Build history of the part. All positions in model axes, mm. Face numbers are marked on the shaded views. A direction names the side the tool comes from. Round coordinates to 2 decimals unless told otherwise and drop trailing zeros. Order: outer loops, then holes, each group sorted by start corner. A loop starts at its lowest first (then second) coordinate and runs counter-clockwise, first axis right, second up. Notation, with made-up numbers: (34.25, -21) - (66.25, -21) arc R14 ccw to (66.25, 6) - close; hole circle Ø3 at (81, 9). An arc over 180 degrees is marked (long way). Write each question's results on one line, items separated by ' | '. Start each with the question number.
```python
from build123d import *
from OCP.BRepFilletAPI import BRepFilletAPI_MakeChamfer

# Parameters (mm, degrees)
BOSS_EXTRUDE1_DEPTH             = 2
BOSS_EXTRUDE2_REACH             = 40.8
SKETCH2_W                       = 18.81765306
SKETCH2_H                       = 6
BOSS_EXTRUDE2_DIRECTION_2_DEPTH = 10
CUT_EXTRUDE1_DEPTH              = 8
CUT_EXTRUDE2_DEPTH              = 38.936459462
CUT_EXTRUDE2_DEPTH_BACK         = 38.936459462
SKETCH4_W                       = 8
SKETCH4_H                       = 2
CHAMFER1_SIZE                   = 2
CHAMFER2_SIZE                   = 10
CHAMFER2_SIZE2                  = 5.773502692
FILLET1_R                       = 20
BOSS_EXTRUDE3_START             = -6
SKETCH5_W                       = 10
SKETCH5_H                       = 1.6
BOSS_EXTRUDE3_DEPTH             = 12


with BuildPart() as part:
    # Sketch1 → Boss-Extrude1 (new, symmetric)
    with BuildSketch(Plane(origin=(0, 0, 0), x_dir=(1, 0, 0), z_dir=(0, 1, 0))):
        Polygon((-8.25, 0), (0, 0), (0, -1.2), (-9.40882653, -1.2), (-9.962319737, 14.649971666), (-19.979363266, 32), (-18.59372262, 32), (-8.773492451, 14.990862405), align=None)
    boss_extrude1 = extrude(amount=BOSS_EXTRUDE1_DEPTH, both=True)

    # Mirror1: Boss-Extrude1 across plane
    add(boss_extrude1.mirror(Plane(origin=(0, 2, 0), x_dir=(0, 0, 1), z_dir=(-1, 0, 0))))

    # Boss-Extrude2: up to this face of the body (flat: up to its plane)
    boss_extrude2_end = Plane(part.part.faces().sort_by_distance((0, 0, 0))[0])
    # Sketch2 → Boss-Extrude2 (add, up to the picked face)
    with BuildSketch(Plane.XY.offset(1.2), mode=Mode.PRIVATE) as boss_extrude2_sk1:
        with Locations((0, -1)):
            Rectangle(SKETCH2_W, SKETCH2_H)
    boss_extrude2_tool1 = split(extrude(boss_extrude2_sk1.sketch, amount=-BOSS_EXTRUDE2_REACH, mode=Mode.PRIVATE), bisect_by=boss_extrude2_end, keep=Keep.BOTH, mode=Mode.PRIVATE)
    add(boss_extrude2_tool1.solids().sort_by(Axis((0, -1, 1.2), (0, 0, -1)))[0])

    # Sketch2 → Boss-Extrude2 direction 2 (add)
    with BuildSketch(Plane.XY.offset(1.2)):
        with Locations((0, -1)):
            Rectangle(SKETCH2_W, SKETCH2_H)
    extrude(amount=BOSS_EXTRUDE2_DIRECTION_2_DEPTH)

    # Sketch3 → Cut-Extrude1 (cut)
    with BuildSketch(Plane.XY.offset(11.2)):
        with BuildLine():
            Line((-1.5, 1.826658805), (-1.5, 2))
            Line((-1.5, 2), (1.5, 2))
            Line((1.5, 2), (1.5, 1.826658805))
            ThreePointArc((1.5, 1.826658805), (3.2, -1), (1.5, -3.826658805))
            Line((1.5, -3.826658805), (1.5, -4))
            Line((1.5, -4), (-1.5, -4))
            Line((-1.5, -4), (-1.5, -3.826658805))
            ThreePointArc((-1.5, -3.826658805), (-3.2, -1), (-1.5, 1.826658805))
        make_face()
    extrude(amount=-CUT_EXTRUDE1_DEPTH, mode=Mode.SUBTRACT)

    # Sketch4 → Cut-Extrude2 (cut, two sides: drawn at the far end of the back side and taken through both)
    with BuildSketch(Plane(origin=(0, 0, 0), x_dir=(1, 0, 0), z_dir=(0, 1, 0)).offset(-CUT_EXTRUDE2_DEPTH_BACK)):
        with Locations((0, -4.2)):
            Rectangle(SKETCH4_W, SKETCH4_H)
    extrude(amount=CUT_EXTRUDE2_DEPTH + CUT_EXTRUDE2_DEPTH_BACK, mode=Mode.SUBTRACT)

    # Chamfer1
    chamfer1_edges = [part.edges().sort_by_distance(p)[0] for p in [
        (8.829413265, -2, 0),
        (-8.829413265, -2, 0),
    ]]
    chamfer(chamfer1_edges, length=CHAMFER1_SIZE - 0.0001)  # a hair under: the kernel refuses the full size

    # Chamfer2: one chamfer whose edges measure the first distance from different faces: ONE call of the kernel's chamfer builder (chamfer() names one face for all edges)
    chamfer2_edges_1 = [part.edges().sort_by_distance(p)[0] for p in [
        (9.40882653, -1, 11.2),
    ]]
    chamfer2_side_1 = [part.faces().sort_by_distance(p)[0] for p in [
        (9.40882653, -1.126288177, 5.77807488),
    ]]
    chamfer2_edges_2 = [part.edges().sort_by_distance(p)[0] for p in [
        (-9.40882653, -1, 11.2),
    ]]
    chamfer2_side_2 = [part.faces().sort_by_distance(p)[0] for p in [
        (-9.40882653, -1.126288177, 5.77807488),
    ]]
    chamfer2 = BRepFilletAPI_MakeChamfer(part.part.solid().wrapped)
    for e in chamfer2_edges_1:
        chamfer2.Add(CHAMFER2_SIZE, CHAMFER2_SIZE2, e.wrapped, chamfer2_side_1[0].wrapped)  # the first distance lies on this face
    for e in chamfer2_edges_2:
        chamfer2.Add(CHAMFER2_SIZE, CHAMFER2_SIZE2, e.wrapped, chamfer2_side_2[0].wrapped)  # the first distance lies on this face
    add(Compound.cast(chamfer2.Shape()), mode=Mode.REPLACE)

    # Fillet1
    fillet1_edges = [part.edges().sort_by_distance(p)[0] for p in [
        (-9.962319737, 0, -14.649971666),
        (-8.773492451, 0, -14.990862405),
        (8.773492451, 0, -14.990862405),
        (9.962319737, 0, -14.649971666),
    ]]
    fillet(fillet1_edges, radius=FILLET1_R)

    # Sketch5 → Boss-Extrude3 (add)
    with BuildSketch(Plane.XZ.offset(4).offset(BOSS_EXTRUDE3_START)):
        with Locations((0, 0.8)):
            Rectangle(SKETCH5_W, SKETCH5_H)
    extrude(amount=BOSS_EXTRUDE3_DEPTH)


solid = part.part
```
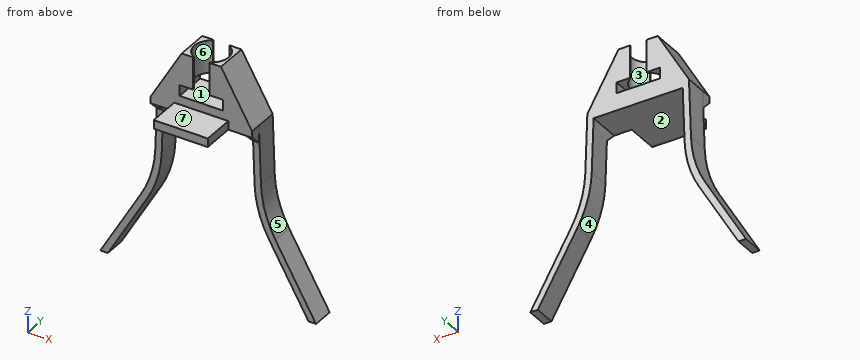
1. 3-axis set-ups, long thin cutter, end or side, ignore diameter. For the marked faces 4, 5, 6 and 7: which of +Z, -Z, +X, -X, +Y, -Y reach the whole face in a straight line?
2. Cut at B-B (x = 0.5). List the corners of the cut face in (y, z), plus the area to 3 significant figures.
3. Flat gauge pins, fed straight in: pin 1 Ø3 at (x, y) = (-2.5, -1.5) entering from -Z; pin 2 Ø8 at (x, z) = (-5, -11.5) entering from -Y; pin 3 Ø0.6 at (y, z) = (-3, 0) entering from -X. Where does each tip first touch, or does it go through?
4. Cut at A-A (z = -13.5). List the corners of the cut face in (x, y).
5. Mould opens along Z. For the marked faces 1, 2 and 3 say: pulls with the +Z half, pulls with the -Z half, needs draft (parallel to the pull), parting line crosses it, or undercut.
6. Cut at D-D (z = -25). List the corners of the cut face in (x, y).
7. Cut at C-C (y = -5.5). List the corners of the cut face in (x, z), plus the area to 3 significant figures.
8. Wall check: line 1 (Z direction, x = 2.5, y = 0.75); line 2 (Y direction, x = 2, z = 7.5); line 3 (X direction, y = 0.25, z = 6). Give the ranges that are in metal, low to high. Write a range as from..to.
A:
1) face 4: -Z, +Y, -Y | face 5: +Z, +X, +Y, -Y | face 6: +Z | face 7: +Z, +X, -X, -Y
2) outline: (-10, 0) - (2, 0) - (2, 3.2) - (-4, 3.2) - (-4, 1.6) - (-10, 1.6) - close | area: 28.8 mm^2
3) pin 1: stops at z = 0 | pin 2: stops at y = -2 | pin 3: stops at x = -9.41
4) outline: (-10.3, -2) - (-9.03, -2) - (-9.03, 2) - (-10.3, 2) - close; (9.03, -2) - (10.3, -2) - (10.3, 2) - (9.03, 2) - close
5) face 1: undercut | face 2: pulls with the -Z half | face 3: needs draft
6) outline: (-15.94, -2) - (-14.55, -2) - (-14.55, 2) - (-15.94, 2) - close; (14.55, -2) - (15.94, -2) - (15.94, 2) - (14.55, 2) - close
7) outline: (-5, 0) - (5, 0) - (5, 1.6) - (-5, 1.6) - close | area: 16.0 mm^2
8) line 1: z = 0..3.2 | line 2: y = -4..-3.5, 1.5..2 | line 3: x = -6.64..-2.95, 2.95..6.64
